```python
from build123d import *

# Parameters (mm, degrees)
F0_W     = 30
F0_H     = 30
F1_DEPTH = 5
F2_R     = 5
F3_SIZE  = 5
F4_T     = -2.5
F6_D     = 5
F8_D     = 5
F8_DEPTH = 15.001


with BuildPart() as f1:
    # F0 (on Front) → F1 (new body, symmetric)
    with BuildSketch(Plane.XZ):
        Rectangle(F0_W, F0_H)
    extrude(amount=F1_DEPTH, both=True)

    # F2
    f2_edges = [f1.edges().sort_by_distance(p)[0] for p in [
        (15, 0, 15),
    ]]
    fillet(f2_edges, radius=F2_R)

    # F3
    f3_edges = [f1.edges().sort_by_distance(p)[0] for p in [
        (15, 0, -15),
    ]]
    chamfer(f3_edges, length=F3_SIZE)

    # F4
    f4_openings = [f1.faces().sort_by_distance(p)[0] for p in [
        (-0.273371, -5, 0.1045),
    ]]
    offset(amount=F4_T, openings=f4_openings)

    # F6 (through all)
    with Locations(Plane.XZ):
        with Locations((0, 0)):
            Hole(F6_D / 2)

    # F8 (through all, one way)
    with BuildSketch(Plane.YZ):
        with Locations((5.0715617836, 5.2282437682)):
            Circle(F8_D / 2)
    extrude(amount=-F8_DEPTH, mode=Mode.SUBTRACT)


solid = f1.part
```
Could you check a few things on this model? Use its own coordinates, in mm. A direction names the side the tool comes from. Round coordinates to 2 decimals unless told otherwise and drop trailing zeros. Loops run counter-clockwise (first coordinate to the right, second up) from the corner with the lowest first, then second, coordinate; pieces in that order, holes last. Notation, with made-up numbers: M -2,-9 L 15,-9 A23 ccw 15,8 Z; hole C 13.5,23.25 d1. An arc over 180 degrees is marked long. Put each result on its own line as item: value.
Q1. Thinking about a two-plate mould opening in X: for faces 4 (the face through (0, 4, 5)), 5 (the face through (0, 2.5, 3)), 6 (the face through (-14, -5, 0)), 7 (the face through (14, 0, 13)), which applies, released by +X, released by -X, zero draft, split by the parting line, or undercut?
Check result:
face 4: released by -X
face 5: undercut
face 6: zero draft
face 7: released by +X
Q2. On a 3-axis mill with a long thin cutter (end or side, diameter ignored), from which of +Z, -Z, +X, -X, +Y, -Y can I reach the whole of each face in a straight line? I mean faces 1 (the face through (-12.5, -1, 0)), 2 (the face through (-7.4, 2.7, 4.44)), 3 (the face through (12, 0, -13)). Say none if no direction works.
Check result:
face 1: -Y
face 2: -X, +Y
face 3: -Z, +X, +Y, -Y
Q3. Imagine slicing it at D-D (z = -6.25). Write out the boundary of the cut face in (x, y).
Check result:
outline: M -15,-5 L -12.5,-5 L -12.5,2.5 L 12.5,2.5 L 12.5,-5 L 15,-5 L 15,5 L -15,5 Z
Q4. Imagine slicing it at C-C (x = -6). Write out the boundary of the cut face in (y, z).
Check result:
outline: M -5,-15 L 5,-15 L 5,2.73 A2.5 cw 5,7.73 L 5,15 L -5,15 L -5,12.5 L 2.5,12.5 L 2.5,-12.5 L -5,-12.5 Z
Q5. I need wall thicknesses on probe 1 along X at (y, z) = (-0.75, 10); probe 2 along Y at (x, z) = (-6.5, -12). Which ranges of each line are inside material? Lowest first, please.
Check result:
probe 1: -15 to -12.5, 12.5 to 15
probe 2: 2.5 to 5
Q6. Imagine slicing it at B-B (z = 0). Write out the boundary of the cut face in (x, y).
Check result:
outline: M -15,-5 L -12.5,-5 L -12.5,2.5 L -2.5,2.5 L -2.5,5 L -15,5 Z; M 2.5,2.5 L 12.5,2.5 L 12.5,-5 L 15,-5 L 15,5 L 2.5,5 Z
Q7. Imagine slicing it at A-A (y = -3). Write out the boundary of the cut face in (x, z).
Check result:
outline: M -15,-15 L 10,-15 L 15,-10 L 15,10 A5 ccw 10,15 L -15,15 Z; hole M -12.5,-12.5 L 8.96,-12.5 L 12.5,-8.96 L 12.5,10 A2.5 ccw 10,12.5 L -12.5,12.5 Z
Q8. For pin 1 (3 mm diameter, centred on x = 8.5, z = 4.5, fed in from -Y); pin 2 (1.9 mm diameter, centred on y = 3.5, z = 5, fed in from -X), each with a flat end and sliding along its axis, tell me the tip position at first contact or that it passes through.
Check result:
pin 1: y = 2.5
pin 2: x = -15
